Answer from the drawing. Dimensions are ordinates in mm from the lowest x, y and z of the part. Give positions to 0.01 mm unless a question says otherwise; leave off trailing zeros. Write each loop counter-clockwise with the first axis right and the second up, starting at its lowest first coordinate (ties: lowest second). Pieces come first, ordered by that corner, then holes.
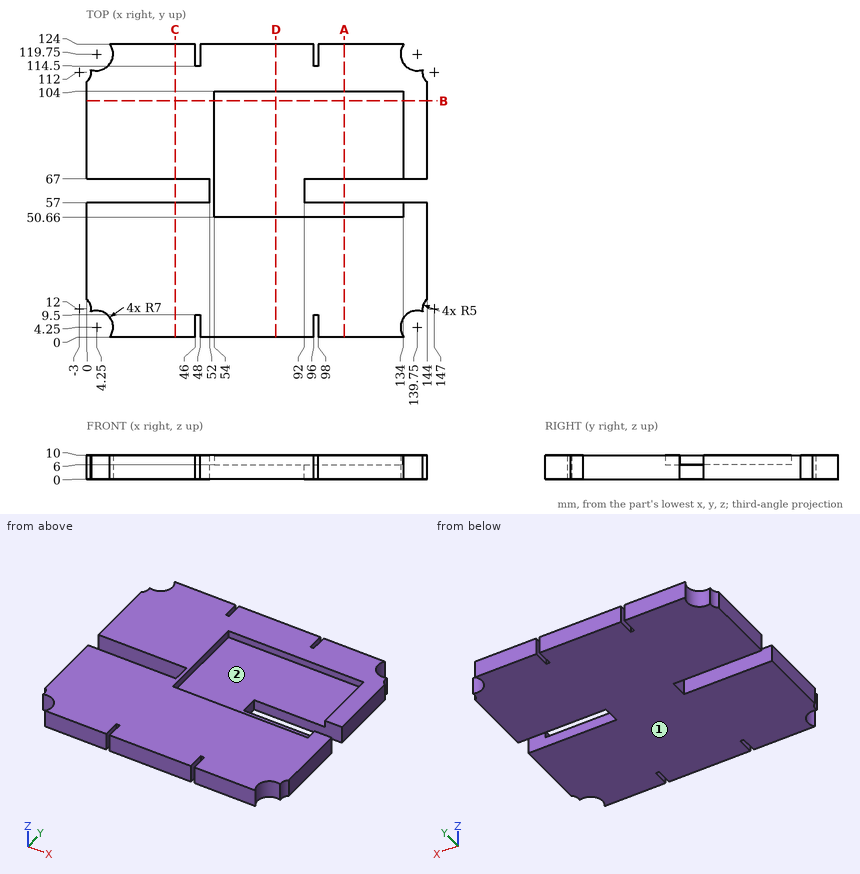
Item 1: Determine the mould class of the marked faces 1 and 2 for opening direction X: pulls with the +X half, pulls with the -X half, needs draft (parallel to the pull), parting line crosses it, or undercut.
Conclusion:
face 1: needs draft
face 2: undercut
Item 2: A cutting plane is placed at A-A, the plane x = 109. Give the vertices of the cut face in (y, z).
Conclusion:
outline: (0, 0) - (57, 0) - (57, 6) - (50.66, 6) - (50.66, 10) - (0, 10) - close; (67, 0) - (124, 0) - (124, 10) - (104, 10) - (104, 6) - (67, 6) - close
Item 3: A cutting plane is placed at D-D, the plane x = 80. Give the vertices of the cut face in (y, z).
Conclusion:
outline: (0, 0) - (124, 0) - (124, 10) - (104, 10) - (104, 6) - (50.66, 6) - (50.66, 10) - (0, 10) - close
Item 4: A cutting plane is placed at B-B, the plane y = 100. Give the vertices of the cut face in (x, z).
Conclusion:
outline: (0, 0) - (144, 0) - (144, 10) - (134, 10) - (134, 6) - (54, 6) - (54, 10) - (0, 10) - close
Item 5: Consider probe 1 along X at (y, z) = (115.5, 5); probe 2 along X at (y, z) = (119.5, 1.5); probe 3 along Y at (x, z) = (75, 7). Determine where each line is inside the solid, lowest interval first.
Conclusion:
probe 1: x = 9.81 to 46, 48 to 96, 98 to 134.19
probe 2: x = 11.25 to 46, 48 to 96, 98 to 132.75
probe 3: y = 0 to 50.66, 104 to 124
Item 6: A cutting plane is placed at C-C, the plane x = 37.5. Give the vertices of the cut face in (y, z).
Conclusion:
outline: (0, 0) - (57, 0) - (57, 10) - (0, 10) - close; (67, 0) - (124, 0) - (124, 10) - (67, 10) - close
Item 7: Each of these flat-tipped pins is pushed along its axis until it touches: P1, Ø3, axis at y = 7, z = 5, coming from the +X side; P2, Ø0.6, axis at x = 46.5, z = 6, coming from the +Y side; P3, Ø3, axis at y = 2.5, z = 3.5, coming from the -X side. Where does it stop, or does it pass through?
Conclusion:
P1: stops at x = 134.19
P2: stops at y = 114.5
P3: stops at x = 10.45
